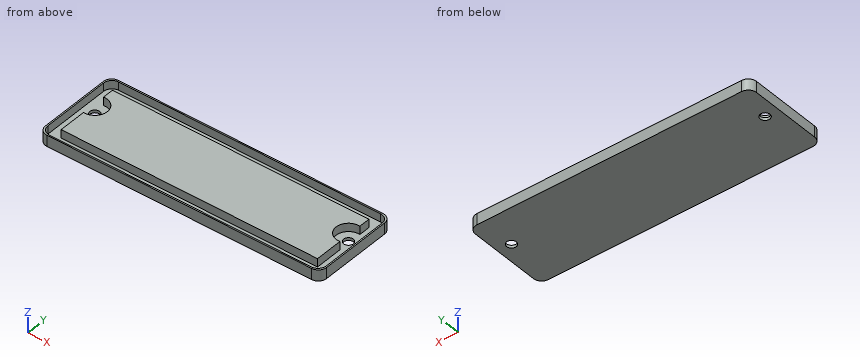
from build123d import *

# Parameters (mm, degrees)
SKETCH1_W           = 102
SKETCH1_H           = 32
BOSS_EXTRUDE1_DEPTH = 1
SKETCH2_W           = 102
SKETCH2_H           = 32
SKETCH2_W_2         = 101
SKETCH2_H_2         = 31
BOSS_EXTRUDE2_DEPTH = 3
SKETCH3_R           = 1.75
CUT_EXTRUDE1_DEPTH  = 107.943910533
FILLET1_R           = 3


with BuildPart() as part:
    # Sketch1 → Boss-Extrude1 (new body)
    with BuildSketch(Plane.XY):
        with Locations((-51, 16)):
            Rectangle(SKETCH1_W, SKETCH1_H)
    extrude(amount=BOSS_EXTRUDE1_DEPTH)

    # Sketch2 → Boss-Extrude2 (add)
    # profile 1 of 2: a face of its own
    with BuildSketch(Plane.XY.offset(1)):
        with Locations((-51, 16)):
            Rectangle(SKETCH2_W, SKETCH2_H)
        with Locations((-51, 16)):
            Rectangle(SKETCH2_W_2, SKETCH2_H_2, mode=Mode.SUBTRACT)
    # profile 2 of 2: a face of its own
    with BuildSketch(Plane.XY.offset(1)):
        with BuildLine():
            Line((-97.5, 14.527864045), (-97.5, 4.5))
            Line((-97.5, 4.5), (-4.5, 4.5))
            Line((-4.5, 4.5), (-4.5, 14.527864045))
            ThreePointArc((-4.5, 14.527864045), (-9.5, 19), (-4.5, 23.472135955))
            Line((-4.5, 23.472135955), (-4.5, 27.5))
            Line((-4.5, 27.5), (-97.5, 27.5))
            Line((-97.5, 27.5), (-97.5, 23.472135955))
            ThreePointArc((-97.5, 23.472135955), (-92.5, 19), (-97.5, 14.527864045))
        make_face()
    extrude(amount=BOSS_EXTRUDE2_DEPTH)

    # Sketch3 → Cut-Extrude1 (cut, through all)
    with BuildSketch(Plane.XY.offset(1)):
        with Locations((-97, 19)):
            Circle(SKETCH3_R)
        with Locations((-5, 19)):
            Circle(SKETCH3_R)
    extrude(amount=-CUT_EXTRUDE1_DEPTH, mode=Mode.SUBTRACT)

    # Fillet1
    fillet1_edges = [part.edges().sort_by_distance(p)[0] for p in [
        (-101.5, 31.5, 2.5),
        (-0.5, 31.5, 2.5),
        (-0.5, 0.5, 2.5),
        (-101.5, 0.5, 2.5),
        (0, 0, 2),
        (-102, 0, 2),
        (-102, 32, 2),
        (0, 32, 2),
    ]]
    fillet(fillet1_edges, radius=FILLET1_R)


solid = part.part
Check sheet for the modelled part. Datum: model origin and axes. Units: mm. Coordinates: 2 decimals unless noted, no trailing zeros. Write each loop counter-clockwise with the first axis right and the second up, starting at its lowest first coordinate (ties: lowest second). Pieces come first, ordered by that corner, then holes.
Item 1: Depth check by flat-ended pin: pin 1 Ø8 at (x, y) = (-5, 19) entering from +Z. Enter the tip coordinate at first touch or a pass-through.
Numbers:
pin 1: stops at z = 1
Item 2: Cross-section at B-B on y = 19. Record the boundary of the cut face in (x, z), then the cut area to 3 significant figures.
Numbers:
outline: (-102, 0) - (-98.75, 0) - (-98.75, 1) - (-101.5, 1) - (-101.5, 4) - (-102, 4) - close; (-95.25, 0) - (-6.75, 0) - (-6.75, 1) - (-9.5, 1) - (-9.5, 4) - (-92.5, 4) - (-92.5, 1) - (-95.25, 1) - close; (-3.25, 0) - (0, 0) - (0, 4) - (-0.5, 4) - (-0.5, 1) - (-3.25, 1) - close
area: 347 mm2
Item 3: Scan lines: probe 1 along X at (y, z) = (19, 2.85); probe 2 along Y at (x, z) = (-67.5, 3.05); probe 3 along Y at (x, z) = (-97, 2.05). Record each from-to range of solid material in increasing order.
Numbers:
probe 1: x = -102 to -101.5, -92.5 to -9.5, -0.5 to 0
probe 2: y = 0 to 0.5, 4.5 to 27.5, 31.5 to 32
probe 3: y = 0 to 0.5, 4.5 to 14.5, 23.5 to 27.5, 31.5 to 32
Item 4: Cross-section at A-A on z = 1.9. Record the boundary of the cut face in (x, y), then the cut area to 3 significant figures.
Numbers:
outline: (-102, 3) arc R3 ccw to (-99, 0) - (-3, 0) arc R3 ccw to (0, 3) - (0, 29) arc R3 ccw to (-3, 32) - (-99, 32) arc R3 ccw to (-102, 29) - close; (-97.5, 4.5) - (-4.5, 4.5) - (-4.5, 14.53) arc R4.5 cw (long way) to (-4.5, 23.47) - (-4.5, 27.5) - (-97.5, 27.5) - (-97.5, 23.47) arc R4.5 cw (long way) to (-97.5, 14.53) - close; hole (-101.5, 3.5) arc R3 ccw to (-98.5, 0.5) - (-3.5, 0.5) arc R3 ccw to (-0.5, 3.5) - (-0.5, 28.5) arc R3 ccw to (-3.5, 31.5) - (-98.5, 31.5) arc R3 ccw to (-101.5, 28.5) - close
area: 2,200 mm2
Item 5: Cross-section at D-D on y = 26.5. Record the boundary of the cut face in (x, z), then the cut area to 3 significant figures.
Numbers:
outline: (-102, 0) - (0, 0) - (0, 4) - (-0.5, 4) - (-0.5, 1) - (-4.5, 1) - (-4.5, 4) - (-97.5, 4) - (-97.5, 1) - (-101.5, 1) - (-101.5, 4) - (-102, 4) - close
area: 384 mm2
Item 6: Cross-section at C-C on x = -20. Record the boundary of the cut face in (y, z).
Numbers:
outline: (0, 0) - (32, 0) - (32, 4) - (31.5, 4) - (31.5, 1) - (27.5, 1) - (27.5, 4) - (4.5, 4) - (4.5, 1) - (0.5, 1) - (0.5, 4) - (0, 4) - close
